Job drawing, mm, ordinate dimensions from the low corner. One solid piece. A direction names the side the tool comes from. Give positions to 0.01 mm unless a question says otherwise; leave off trailing zeros. Order: outer loops, then holes, each group sorted by start corner. A loop starts at its lowest first (then second) coordinate and runs counter-clockwise, first axis right, second up. Notation, with made-up numbers: (36.25, 52.25) - (49.25, 52.25) arc R27 cw to (49.25, 81.25) - close; hole circle Ø10 at (75, 41). An arc over 180 degrees is marked (long way). One line per item, written item: value.
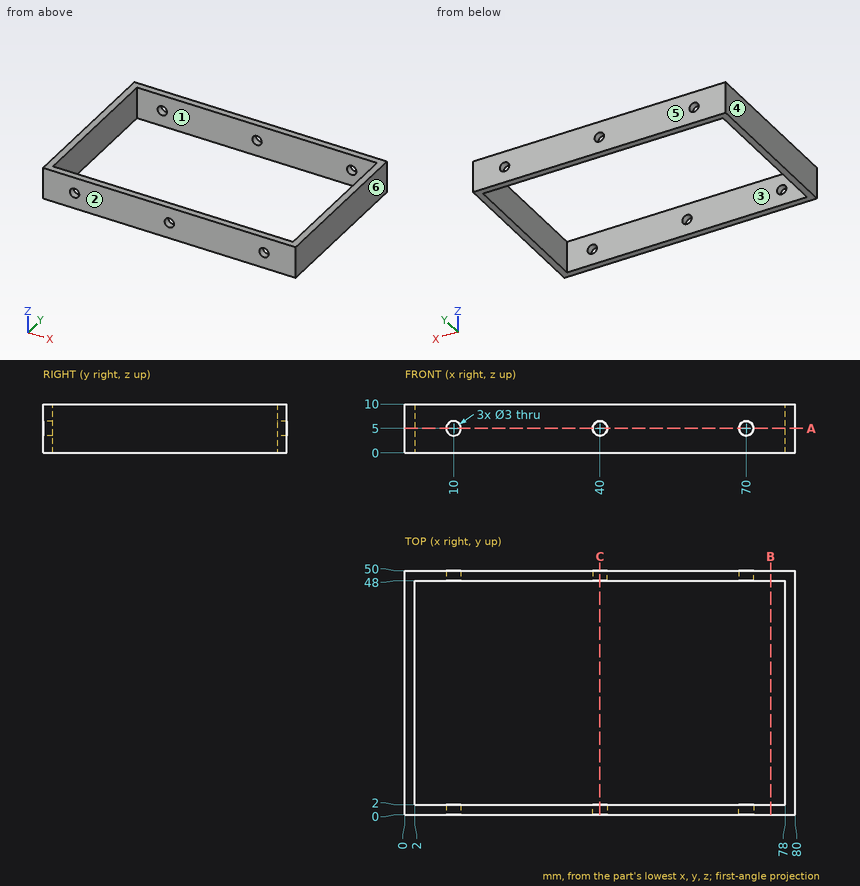
1) Slice it at A-A on z = 5. Count the separate pieces of the cut face and the enclosed holes in it, then the cut area to 3 significant figures.
Answer:
separate pieces: 6
enclosed holes: 0
area: 468 mm2
2) Wall check: line 1 along X through (y, z) = (46, 5.75); line 2 along Y through (x, z) = (64.5, 4.5); line 3 along Z through (x, y) = (10, 48.9). Give the ranges that are in metal, low to high. Write a range as [from, to].
Answer:
line 1: x = [0, 2], [78, 80]
line 2: y = [0, 2], [48, 50]
line 3: z = [0, 3.5], [6.5, 10]
3) Which spindle directions (+Z, -Z, +X, -X, +Y, -Y) get a long thin tool onto all of the face, cutting with end or side? Do the marked faces 1 and 2. Say none if no direction does.
Answer:
face 1: +Z, -Z
face 2: +Z, -Z, +X, -X, -Y
4) Slice it at B-B on x = 75. Write the cut outline in (y, z), then the cut area to 3 significant figures.
Answer:
outline: (0, 0) - (2, 0) - (2, 10) - (0, 10) - close; (48, 0) - (50, 0) - (50, 10) - (48, 10) - close
area: 40.0 mm2
5) Slice it at C-C on x = 40. Write the cut outline in (y, z).
Answer:
outline: (0, 0) - (2, 0) - (2, 3.5) - (0, 3.5) - close; (0, 6.5) - (2, 6.5) - (2, 10) - (0, 10) - close; (48, 0) - (50, 0) - (50, 3.5) - (48, 3.5) - close; (48, 6.5) - (50, 6.5) - (50, 10) - (48, 10) - close
6) Two-plate mould, pull along X, no slides. Class the marked faces 3, 4, 5 and 6: pulls with the +X half, pulls with the -X half, needs draft (parallel to the pull), parting line crosses it, or undercut.
Answer:
face 3: undercut
face 4: pulls with the -X half
face 5: needs draft
face 6: pulls with the +X half
